from build123d import *

# Parameters (mm, degrees)
SKETCH_1_W            = 42
SKETCH_1_H            = 25.4
EXTRUDE_1_DEPTH       = 70
SKETCH_5_W            = 6
SKETCH_5_H            = 25.4
EXTRUDE_5_DEPTH       = 70
SKETCH_6_R            = 4.7625
CUT_EXTRUDE_2_DEPTH   = 83.61531335
FILLET_6_R            = 4
HOLE_WIZARD_10_32_1_D = 4.0386
FILLET_7_R            = 12.7
SKETCH_9_W            = 42
SKETCH_9_H            = 25
CUT_EXTRUDE_3_DEPTH   = 78.370278531
HOLE_WIZARD_10_32_2_D = 4.0386


with BuildPart() as part:
    # 草圖1 → 填料-伸長1 (new body)
    with BuildSketch(Plane(origin=(0, 0, 0), x_dir=(1, 0, 0), z_dir=(0, 1, 0))):
        Rectangle(SKETCH_1_W, SKETCH_1_H)
    extrude(amount=EXTRUDE_1_DEPTH)

    # 草圖5 → 填料-伸長5 (add)
    with BuildSketch(Plane.XZ):
        with Locations((-18, 0)):
            Rectangle(SKETCH_5_W, SKETCH_5_H)
        with Locations((18, 0)):
            Rectangle(SKETCH_5_W, SKETCH_5_H)
    extrude(amount=EXTRUDE_5_DEPTH)

    # 草圖6 → 除料-伸長2 (cut, through all)
    with BuildSketch(Plane.ZY.offset(21)):
        with Locations((0, -57.3)):
            Circle(SKETCH_6_R)
    extrude(amount=-CUT_EXTRUDE_2_DEPTH, mode=Mode.SUBTRACT)

    # 圓角6
    fillet_6_edges = [part.edges().sort_by_distance(p)[0] for p in [
        (15, 0, 0),
        (-15, 0, 0),
    ]]
    fillet(fillet_6_edges, radius=FILLET_6_R)

    # #10-32 螺紋孔1 (through all)
    with Locations(Plane.XY.offset(12.7)):
        with Locations((0, 30), (0, 15)):
            Hole(HOLE_WIZARD_10_32_1_D / 2)

    # 圓角7
    fillet_7_edges = [part.edges().sort_by_distance(p)[0] for p in [
        (18, -70, 12.7),
        (18, -70, -12.7),
        (-18, -70, 12.7),
        (-18, -70, -12.7),
    ]]
    fillet(fillet_7_edges, radius=FILLET_7_R - 0.0001)  # a hair under: the kernel refuses the full size

    # 草圖9 → 除料-伸長3 (cut, through all)
    with BuildSketch(Plane.XY.offset(12.7)):
        with Locations((0, 57.5)):
            Rectangle(SKETCH_9_W, SKETCH_9_H)
    extrude(amount=-CUT_EXTRUDE_3_DEPTH, mode=Mode.SUBTRACT)

    # #10-32 螺紋孔2 (through all)
    with Locations(Plane(origin=(21, 0, 0), x_dir=(0, 0, -1), z_dir=(1, 0, 0))):
        with Locations((0, -11.3), (0, -19.3), (0, -27.3)):
            Hole(HOLE_WIZARD_10_32_2_D / 2)


solid = part.part
Design review of the part built by this model. Coordinates are the model's own, in mm. A direction names the side the tool comes from. Round coordinates to 2 decimals unless told otherwise and drop trailing zeros. Write each loop counter-clockwise with the first axis right and the second up, starting at its lowest first coordinate (ties: lowest second). Pieces come first, ordered by that corner, then holes. Notation, with made-up numbers: (-37, -28) -> (-22, -28) arc R35 ccw to (-22, 5) -> close; hole circle Ø1 at (-32, 29). An arc over 180 degrees is marked (long way). One line per item, written item: value. Start each with the question number.
Q1. Insertion check: P1, Ø12, axis at x = 9.5, z = 5, coming from the -Y side; P2, Ø5.5, axis at y = -57.3, z = 0, coming from the -X side; P3, Ø11, axis at x = 3.5, z = -0.5, coming from the -Y side; P4, Ø6, axis at x = 10, z = -3, coming from the -Y side. Each pin has a flat end and moves straight along its axis. Give the tip position at first contact, or say it passes through.
Q2. Add section D-D (y = -27.3). Give the boundary of the cut face in (x, z), then the cut area to 3 significant figures.
Q3. Add section B-B (x = 0). Give the boundary of the cut face in (y, z).
Q4. Add section A-A (y = 15). Give the boundary of the cut face in (x, z), then the cut area to 3 significant figures.
Q5. Add section C-C (z = -3.75). Give the boundary of the cut face in (x, y), then the cut area to 3 significant figures.
Q6. To check wall thickness, follow probe 1 along Y at (x, z) = (-18.35, 0); probe 2 along Y at (x, z) = (0, -6.25); probe 3 along Z at (x, y) = (19, -27). State the ranges of each line that lie inside material, in increasing order.
Q7. Tool access review of faces 4 (the face through (-21, -12, 3)), 5 (the face through (-13.859, -1.203, 0.178)): name each direction out of +Z, -Z, +X, -X, +Y, -Y from which nothing blocks a thin tool from reaching the whole face with its end or side.
Q8. The part is to be moulded in two halves that separate along Y. For faces 1 (the face through (15, -37, 0)), 2 (the face through (0, 0, 0)), 3 (the face through (-18.04, -54.08, -3.51)), say which applies: pulls with the +Y half, pulls with the -Y half, needs draft (parallel to the pull), parting line crosses it, or undercut.
Response:
1. P1: stops at y = -69.73
1. P2: passes through
1. P3: stops at y = 0
1. P4: stops at y = -0.54
2. outline: (-21, -12.7) -> (-15, -12.7) -> (-15, -2.02) -> (-21, -2.02) -> close; (-21, 2.02) -> (-15, 2.02) -> (-15, 12.7) -> (-21, 12.7) -> close; (15, -12.7) -> (21, -12.7) -> (21, -2.02) -> (15, -2.02) -> close; (15, 2.02) -> (21, 2.02) -> (21, 12.7) -> (15, 12.7) -> close
2. area: 256 mm^2
3. outline: (0, -12.7) -> (12.98, -12.7) -> (12.98, 12.7) -> (0, 12.7) -> close; (17.02, -12.7) -> (27.98, -12.7) -> (27.98, 12.7) -> (17.02, 12.7) -> close; (32.02, -12.7) -> (45, -12.7) -> (45, 12.7) -> (32.02, 12.7) -> close
4. outline: (-21, -12.7) -> (-2.02, -12.7) -> (-2.02, 12.7) -> (-21, 12.7) -> close; (2.02, -12.7) -> (21, -12.7) -> (21, 12.7) -> (2.02, 12.7) -> close
4. area: 964 mm^2
5. outline: (-21, -69.43) -> (-15, -69.43) -> (-15, -60.24) -> (-21, -60.24) -> close; (-21, -54.36) -> (-15, -54.36) -> (-15, -4) arc R4 cw to (-11, 0) -> (11, 0) arc R4 cw to (15, -4) -> (15, -54.36) -> (21, -54.36) -> (21, 45) -> (-21, 45) -> close; (15, -69.43) -> (21, -69.43) -> (21, -60.24) -> (15, -60.24) -> close; hole circle Ø4.04 at (0, 15); hole circle Ø4.04 at (0, 30)
5. area: 2,630 mm^2
6. probe 1: y = -70 to -62.06, -52.54 to -29.32, -25.28 to -21.32, -17.28 to -13.32, -9.28 to 45
6. probe 2: y = 0 to 12.98, 17.02 to 27.98, 32.02 to 45
6. probe 3: z = -12.7 to -2, 2 to 12.7
7. face 4: +Z, -Z, -X, +Y, -Y
7. face 5: +Z, -Z, -Y
8. face 1: needs draft
8. face 2: pulls with the -Y half
8. face 3: undercut
